from build123d import *

# Parameters (mm, degrees)
BOSS_EXTRU_1_DEPTH           = 345
ENL_V_MAT_EXTRU_1_DEPTH      = 421.149973224
ENL_V_MAT_EXTRU_1_DEPTH_BACK = 421.149973224
ESQUISSE5_W                  = 400
ESQUISSE5_H                  = 70
ENL_V_MAT_EXTRU_3_DEPTH      = 75
ESQUISSE6_W                  = 20
ESQUISSE6_H                  = 21
ENL_V_MAT_EXTRU_4_DEPTH      = 1


with BuildPart() as part:
    # Esquisse1 → Boss.-Extru.1 (new body)
    with BuildSketch(Plane(origin=(0, 0, 0), x_dir=(1, 0, 0), z_dir=(0, 1, 0))):
        with BuildLine():
            Line((-165, -55.235857919), (-165, 55.235857919))
            ThreePointArc((-165, 55.235857919), (0, 174), (165, 55.235857919))
            Line((165, 55.235857919), (165, -55.235857919))
            ThreePointArc((165, -55.235857919), (127.908511428, -117.963607542), (68.381283989, -160))
            Line((68.381283989, -160), (-68.381283989, -160))
            ThreePointArc((-68.381283989, -160), (-127.908511428, -117.963607542), (-165, -55.235857919))
        make_face()
    extrude(amount=BOSS_EXTRU_1_DEPTH)

    # Esquisse3 → Enlèv. mat.-Extru.1 (cut, two sides: drawn at the far end of the back side and taken through both)
    with BuildSketch(Plane.ZY.offset(-ENL_V_MAT_EXTRU_1_DEPTH_BACK)):
        Polygon((-50, 345), (-542.711062326, 0), (-542.711062326, 345), align=None)
        Polygon((-60, 150), (-130, 150), (-130, 75), (-150, 75), (-150, 0), (-174, 0), (-174, 235), (-60, 235), align=None)
    extrude(amount=ENL_V_MAT_EXTRU_1_DEPTH + ENL_V_MAT_EXTRU_1_DEPTH_BACK, mode=Mode.SUBTRACT)

    # Esquisse5 → Enlèv. mat.-Extru.3 (cut)
    with BuildSketch(Plane(origin=(0, 150, 0), x_dir=(1, 0, 0), z_dir=(0, 1, 0))):
        with Locations((0, 95)):
            Rectangle(ESQUISSE5_W, ESQUISSE5_H)
    extrude(amount=-ENL_V_MAT_EXTRU_3_DEPTH, mode=Mode.SUBTRACT)

    # Esquisse6 → Enlèv. mat.-Extru.4 (cut)
    with BuildSketch(Plane.XZ):
        with Locations((0, 149.5)):
            Rectangle(ESQUISSE6_W, ESQUISSE6_H)
    extrude(amount=-ENL_V_MAT_EXTRU_4_DEPTH, mode=Mode.SUBTRACT)


solid = part.part
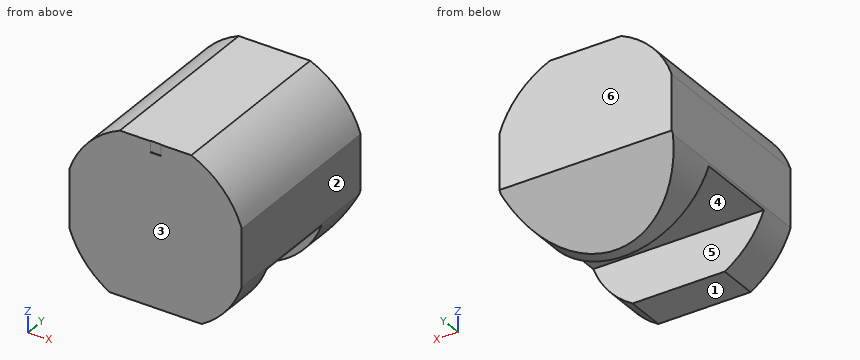
Verification items for the finished model (mm, model axes). Face numbers are marked on the shaded views. A direction names the side the tool comes from. Round coordinates to 2 decimals unless told otherwise and drop trailing zeros. Loops run counter-clockwise (first coordinate to the right, second up) from the corner with the lowest first, then second, coordinate; pieces in that order, holes last. Notation, with made-up numbers: (33, 89) - (56, 89) arc R12 cw to (56, 93) - close; hole circle Ø3 at (42.5, 58). An arc over 180 degrees is marked (long way). Use a Markdown table: item, result. Add a question column.
1. Gauge pin test, flat ends, axial feed: pin 1 (3 mm diameter, centred on x = 84.5, y = 201.5, fed in from -Z); pin 2 (0.8 mm diameter, centred on y = 0.5, z = 146.5, fed in from +X); pin 3 (6 mm diameter, centred on x = -4.5, z = 153.5, fed in from -Y). Record the tip position at first contact, or that the pin passes through.
2. Section check A-A, the plane y = 250.5. Record the boundary of the cut face in (x, z), plus the area to 3 significant figures.
3. Access from +Z, -Z, +X, -X, +Y, -Y to the whole of each face (thin tool, end or side, straight path). Record for the marked faces 1 and 2.
4. Section check B-B, the plane x = 109.5. Record the boundary of the cut face in (y, z).
5. Thickness scan on probe 1 along Z at (x, y) = (150, 261.5); probe 2 along Z at (x, y) = (12.5, 164); probe 3 along Y at (x, z) = (71.5, -105). Record the ranges inside material, lowest first. Write a range as [from, to].
6. Section check D-D, the plane z = 126. Record the boundary of the cut face in (x, y).
7. Release check for a two-part mould opening along Y. For the marked faces 3, 4, 5 and 6 record: released by +Y, released by -Y, zero draft, split by the parting line, or undercut.
8. Section check C-C, the plane y = 139.5. Record the boundary of the cut face in (x, z), plus the area to 3 significant figures.
Checks:
| question | item | result |
|---|---|---|
| 1 | pin 1 | stops at z = -60 |
| 1 | pin 2 | stops at x = 94.5 |
| 1 | pin 3 | stops at y = 1 |
| 2 | outline | (-165, -55.24) arc R174 ccw to (165, -55.24) - (165, 55.24) arc R174 ccw to (68.38, 160) - (-68.38, 160) arc R174 ccw to (-165, 55.24) - close |
| 2 | area | 92,500 mm^2 |
| 3 | face 1 | -Z, +X, -X, -Y |
| 3 | face 2 | +Z, -Z, +X, +Y, -Y |
| 4 | outline | (0, -135.22) - (75, -135.22) - (75, -60) - (235, -60) - (235, -135.22) - (285.32, -135.22) - (345, -50) - (345, 135.22) - (0, 135.22) - close |
| 5 | probe 1 | z = [-88.18, 88.18] |
| 5 | probe 2 | z = [-60, 160] |
| 5 | probe 3 | y = [0, 75], [235, 306.49] |
| 6 | outline | (-120, 0) - (120, 0) - (120, 345) - (-120, 345) - close |
| 7 | face 3 | released by -Y |
| 7 | face 4 | undercut |
| 7 | face 5 | undercut |
| 7 | face 6 | released by +Y |
| 8 | outline | (-165, -55.24) arc R174 ccw to (-163.33, -60) - (163.33, -60) arc R174 ccw to (165, -55.24) - (165, 55.24) arc R174 ccw to (68.38, 160) - (-68.38, 160) arc R174 ccw to (-165, 55.24) - close |
| 8 | area | 65,400 mm^2 |
